Geometry check sheet. Reference: the model listing, model coordinates, mm. A direction names the side the tool comes from. Coordinates: 2 decimals unless noted, no trailing zeros. Order: outer loops, then holes, each group sorted by start corner. A loop starts at its lowest first (then second) coordinate and runs counter-clockwise, first axis right, second up. Notation, with made-up numbers: (86.25, 44.5) - (131.25, 44.5) arc R23 ccw to (131.25, 61.5) - close; hole circle Ø4 at (81.25, -15.75). An arc over 180 degrees is marked (long way). Put each result on its own line as item: value.
from build123d import *

# Parameters (mm, degrees)
SWEEP1_PROFILE_R     = 9.9375
CUT_SWEEP1_PROFILE_R = 7.9375
SWEEP2_PROFILE_R     = 11.525
CUT_SWEEP2_PROFILE_R = 9.525


with BuildPart() as part:
    # Sweep1: sweep along a path in Sketch9
    with BuildLine(Plane(origin=(0, 0, 0), x_dir=(1, 0, 0), z_dir=(0, 1, 0))) as sweep1_path:
        Line((0, 0), (0, 31.75))
    # Sweep1 profile (on start of the path) → Sweep1 (sweep)
    with BuildSketch(Plane(origin=(0, 0, 0), x_dir=(-1, 0, 0), z_dir=(0, 0, -1))):
        Circle(SWEEP1_PROFILE_R)
    sweep(path=sweep1_path.line)

    # Cut-Sweep1: sweep along a path in Sketch9<2>
    with BuildLine(Plane(origin=(0, 0, 0), x_dir=(1, 0, 0), z_dir=(0, 1, 0))) as cut_sweep1_path:
        Line((0, 0), (0, 31.75))
    # Cut-Sweep1 profile (on start of the path) → Cut-Sweep1 (sweep, cut)
    with BuildSketch(Plane(origin=(0, 0, 0), x_dir=(-1, 0, 0), z_dir=(0, 0, -1))):
        Circle(CUT_SWEEP1_PROFILE_R)
    sweep(path=cut_sweep1_path.line, mode=Mode.SUBTRACT)

    # Sweep2: sweep along a path in Sketch31
    with BuildLine(Plane(origin=(0, 0, 0), x_dir=(1, 0, 0), z_dir=(0, 1, 0))) as sweep2_path:
        Line((0, 31.75), (0, 104.0384))
    # Sweep2 profile (on start of the path) → Sweep2 (sweep)
    with BuildSketch(Plane(origin=(0, 0, -31.75), x_dir=(-1, 0, 0), z_dir=(0, 0, -1))):
        Circle(SWEEP2_PROFILE_R)
    sweep(path=sweep2_path.line)

    # Cut-Sweep2: sweep along a path in Sketch31<2>
    with BuildLine(Plane(origin=(0, 0, 0), x_dir=(1, 0, 0), z_dir=(0, 1, 0))) as cut_sweep2_path:
        Line((0, 31.75), (0, 104.0384))
    # Cut-Sweep2 profile (on start of the path) → Cut-Sweep2 (sweep, cut)
    with BuildSketch(Plane(origin=(0, 0, -31.75), x_dir=(-1, 0, 0), z_dir=(0, 0, -1))):
        Circle(CUT_SWEEP2_PROFILE_R)
    sweep(path=cut_sweep2_path.line, mode=Mode.SUBTRACT)


solid = part.part
Q1. Access from +Z, -Z, +X, -X, +Y, -Y to the whole of each face (thin tool, end or side, straight path). Record for faces 1 (the flat face through (-5, 9, -31.75)), 2 (the flat face through (2, 8, -31.75)), 3 (the cylindrical face through (8.494, 7.789, -68.4)).
Answer block:
face 1: +Z
face 2: -Z
face 3: +Z, -Z
Q2. Section check D-D on z = -62. Record the boundary of the cut face in (x, y) (3 decimals), then the cut area to 3 significant figures.
Answer block:
outline: circle Ø23.05 at (0, 0); hole circle Ø19.05 at (0, 0)
area: 132 mm^2
Q3. Draft check along Y on faces 4 (the cylindrical face through (1.72, -7.75, -16.1)), 5 (the flat face through (4, 9, -104.038)), 6 (the cylindrical face through (1.294, 9.853, -16.097)). Enter one of: pulls with the +Y half, pulls with the -Y half, needs draft (parallel to the pull), parting line crosses it, or undercut.
Answer block:
face 4: undercut
face 5: needs draft
face 6: parting line crosses it
Q4. Depth check by flat-ended pin: pin 1 Ø6 at (x, z) = (-4, -29) entering from -Y; pin 2 Ø4 at (x, z) = (1.5, -19.5) entering from -Y; pin 3 Ø1 at (x, z) = (1.5, -35) entering from +Y; pin 4 Ø1 at (x, y) = (6.5, -3) entering from -Z. Enter the tip coordinate at first touch or a pass-through.
Answer block:
pin 1: stops at y = -11.18
pin 2: stops at y = -9.94
pin 3: stops at y = 11.48
pin 4: passes through
Q5. Thickness scan on L1, parallel to Y at x = 0.25, z = -32.5; L2, parallel to Z at x = -8, y = 1.25; L3, parallel to Z at x = -10.5, y = 0.5. Record the ranges inside material, lowest first. Write a range as [from, to].
Answer block:
L1: y = [-11.52, -9.52], [9.52, 11.52]
L2: z = [-31.75, 0]
L3: z = [-104.04, -31.75]
Q6. Section check C-C on z = -12. Record the boundary of the cut face in (x, y) (1 decimal), then the cut area to 3 significant figures.
Answer block:
outline: circle Ø19.9 at (0, 0); hole circle Ø15.9 at (0, 0)
area: 112 mm^2
